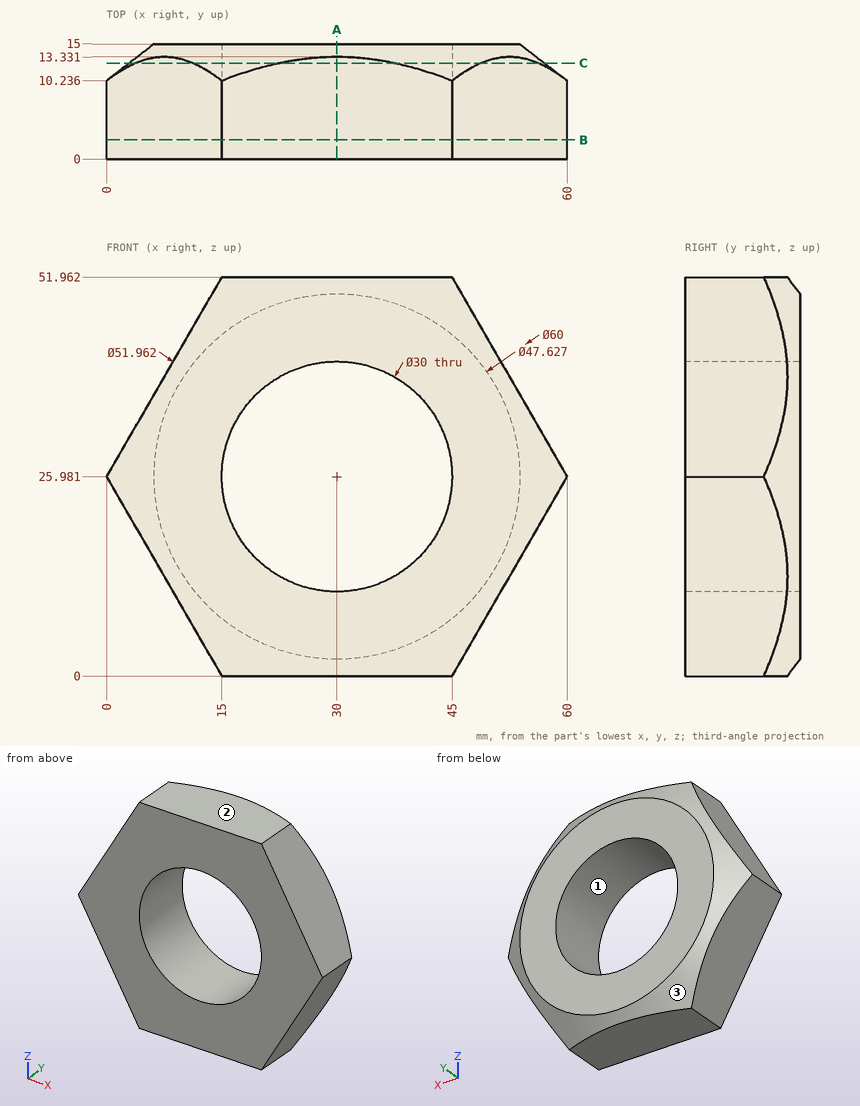
For this review, use the dimensioned drawing (mm, ordinates from the lowest corner) and the shaded views. Give positions to 0.01 mm unless a question says otherwise; leave off trailing zeros. Write each loop counter-clockwise with the first axis right and the second up, starting at its lowest first coordinate (ties: lowest second). Pieces come first, ordered by that corner, then holes.
(1) The part is to be moulded in two halves that separate along X. For the marked faces 1, 2 and 3, say which applies: released by +X, released by -X, zero draft, split by the parting line, or undercut.
(2) To check wall thickness, follow L1, parallel to X at y = 9.75, z = 14 (1 decimal); L2, parallel to X at y = 4, z = 17 (1 decimal); L3, parallel to Z at x = 29.5, y = 5. State the ranges of each line that lie inside material, in increasing order.
(3) For P1, Ø2, axis at x = 9, y = 5, coming from the +Z side; P2, Ø6, axis at y = 13, z = 32, coming from the +X side; P3, Ø1, axis at x = 46.5, y = 3, coming from the -Z side (1 decimal), all flat-tipped, find the tip position at first contact; note any pin that passes through.
(4) Consider section B-B, the plane y = 2.5. Give the boundary of the cut face in (x, z), and give its area (3 significant figures).
(5) Consider section C-C, the plane y = 12.5. Give the boundary of the cut face in (x, z).
(6) Consider section A-A, the plane x = 30. Give the boundary of the cut face in (y, z) (1 decimal), and give its area (3 significant figures).
Returned:
1. face 1: undercut
1. face 2: zero draft
1. face 3: split by the parting line
2. L1: x = 6.9 to 21, 39 to 53.1
2. L2: x = 5.2 to 18, 42 to 54.8
2. L3: z = 0 to 10.99, 40.97 to 51.96
3. P1: stops at z = 43.3
3. P2: stops at x = 58.05
3. P3: stops at z = 1.7
4. outline: (0, 25.98) - (15, 0) - (45, 0) - (60, 25.98) - (45, 51.96) - (15, 51.96) - close; hole circle Ø30 at (30, 25.98)
4. area: 1,630 mm2
5. outline: (3.72, 19.54) - (11.28, 6.44) arc R27.06 ccw to (22.43, 0) - (37.57, 0) arc R27.06 ccw to (48.72, 6.44) - (56.28, 19.54) arc R27.06 ccw to (56.28, 32.42) - (48.72, 45.52) arc R27.06 ccw to (37.57, 51.96) - (22.43, 51.96) arc R27.06 ccw to (11.28, 45.52) - (3.72, 32.42) arc R27.06 ccw to start; hole circle Ø30 at (30, 25.98)
6. outline: (0, 0) - (13.3, 0) - (15, 2.2) - (15, 11) - (0, 11) - close; (0, 41) - (15, 41) - (15, 49.8) - (13.3, 52) - (0, 52) - close
6. area: 326 mm2
